The model under review builds one solid part; all positions refer to its coordinate system, in mm. Round coordinates to 2 decimals unless told otherwise and drop trailing zeros. Order: outer loops, then holes, each group sorted by start corner. A loop starts at its lowest first (then second) coordinate and runs counter-clockwise, first axis right, second up.
```python
from build123d import *

# Parameters (mm, degrees)
SKETCH1_W                                            = 150
SKETCH1_H                                            = 65
BOSS_EXTRUDE1_DEPTH                                  = 3
SKETCH2_W                                            = 130
SKETCH2_H                                            = 45
CUT_EXTRUDE1_DEPTH                                   = 82.793948431
FILLET1_R                                            = 2
SKETCH3_W                                            = 145
SKETCH3_H                                            = 60
CUT_EXTRUDE2_DEPTH                                   = 0.6
FILLET2_R                                            = 2
CSK_FOR_M2_5_CROSS_RECESSED_CTSK_HEAD_WO_D           = 2.7
CSK_FOR_M2_5_CROSS_RECESSED_CTSK_HEAD_WO_CSINK_D     = 5.4
CSK_FOR_M2_5_CROSS_RECESSED_CTSK_HEAD_WO_CSINK_ANGLE = 90
CHAMFER1_SIZE                                        = 1


with BuildPart() as part:
    # Sketch1 → Boss-Extrude1 (new body)
    with BuildSketch(Plane.XY):
        Rectangle(SKETCH1_W, SKETCH1_H)
    extrude(amount=BOSS_EXTRUDE1_DEPTH)

    # Sketch2 → Cut-Extrude1 (cut, through all)
    with BuildSketch(Plane.XY.offset(3)):
        Rectangle(SKETCH2_W, SKETCH2_H)
    extrude(amount=-CUT_EXTRUDE1_DEPTH, mode=Mode.SUBTRACT)

    # Fillet1
    fillet1_edges = [part.edges().sort_by_distance(p)[0] for p in [
        (-65, -22.5, 1.5),
        (-65, 22.5, 1.5),
        (65, 22.5, 1.5),
        (65, -22.5, 1.5),
        (-75, 32.5, 1.5),
        (75, 32.5, 1.5),
        (75, -32.5, 1.5),
        (-75, -32.5, 1.5),
    ]]
    fillet(fillet1_edges, radius=FILLET1_R)

    # Sketch3 → Cut-Extrude2 (cut)
    with BuildSketch(Plane.XY):
        Rectangle(SKETCH3_W, SKETCH3_H)
    extrude(amount=CUT_EXTRUDE2_DEPTH, mode=Mode.SUBTRACT)

    # Fillet2
    fillet2_edges = [part.edges().sort_by_distance(p)[0] for p in [
        (-72.5, 30, 0.3),
        (-72.5, -30, 0.3),
        (72.5, -30, 0.3),
        (72.5, 30, 0.3),
    ]]
    fillet(fillet2_edges, radius=FILLET2_R)

    # CSK for M2.5 Cross recessed CTSK head wood screws1 (through all)
    with Locations(Plane.XY.offset(3)):
        with Locations((-70, 27.5), (-70, 17.5), (-70, 5.833333333), (-70, -5.833333333), (-70, -17.5), (-70, -27.5), (-60, 27.5), (-42.857142857, 27.5), (-25.714285714, 27.5), (-8.571428571, 27.5), (8.571428571, 27.5), (25.714285714, 27.5), (42.857142857, 27.5), (60, 27.5), (70, 27.5), (70, 17.5), (70, 5.833333333), (70, -5.833333333), (70, -17.5), (70, -27.5), (60, -27.5), (42.857142857, -27.5), (25.714285714, -27.5), (8.571428571, -27.5), (-8.571428571, -27.5), (-25.714285714, -27.5), (-42.857142857, -27.5), (-60, -27.5)):
            CounterSinkHole(CSK_FOR_M2_5_CROSS_RECESSED_CTSK_HEAD_WO_D / 2, CSK_FOR_M2_5_CROSS_RECESSED_CTSK_HEAD_WO_CSINK_D / 2, counter_sink_angle=CSK_FOR_M2_5_CROSS_RECESSED_CTSK_HEAD_WO_CSINK_ANGLE)

    # Chamfer1
    chamfer1_edges = [part.edges().sort_by_distance(p)[0] for p in [
        (0, 32.5, 3),
        (75, 0, 3),
        (-75, 0, 3),
        (0, -32.5, 3),
        (-74.414213562, 31.914213562, 3),
        (-74.414213562, -31.914213562, 3),
        (74.414213562, -31.914213562, 3),
        (74.414213562, 31.914213562, 3),
    ]]
    chamfer(chamfer1_edges, length=CHAMFER1_SIZE)


solid = part.part
```
(1) To check wall thickness, follow probe 1 along X at (y, z) = (-17.5, 1.55); probe 2 along Y at (x, z) = (-25.5, 1.7); probe 3 along Y at (x, z) = (-43, 1.5). State the ranges of each line that lie inside material, in increasing order.
Data:
probe 1: x = -75 to -71.35, -68.65 to -65, 65 to 68.65, 71.35 to 75
probe 2: y = -32.5 to -28.88, -26.12 to -22.5, 22.5 to 26.12, 28.88 to 32.5
probe 3: y = -32.5 to -28.84, -26.16 to -22.5, 22.5 to 26.16, 28.84 to 32.5
(2) Draft analysis for pull direction X (two halves, no side actions). For faces 1 (the cylindrical face through (-43.48, -28.698, 1.118)), 2 (the cylindrical face through (69.38, 26.3, 1.12)), 3 (the flat face through (-6, 23, 3)), state which applies: pulls with the +X half, pulls with the -X half, needs draft (parallel to the pull), parting line crosses it, or undercut.
Data:
face 1: undercut
face 2: undercut
face 3: needs draft
(3) Consider section B-B (x = 60). Write out the cut boundary in (y, z).
Data:
outline: (-32.5, 0) - (-30, 0) - (-30, 0.6) - (-28.85, 0.6) - (-28.85, 1.65) - (-30.2, 3) - (-31.5, 3) - (-32.5, 2) - close; (-26.15, 0.6) - (-22.5, 0.6) - (-22.5, 3) - (-24.8, 3) - (-26.15, 1.65) - close; (22.5, 0.6) - (26.15, 0.6) - (26.15, 1.65) - (24.8, 3) - (22.5, 3) - close; (28.85, 0.6) - (30, 0.6) - (30, 0) - (32.5, 0) - (32.5, 2) - (31.5, 3) - (30.2, 3) - (28.85, 1.65) - close
(4) Consider section D-D (x = -31). Write out the cut boundary in (y, z), and give its area (3 significant figures).
Data:
outline: (-32.5, 0) - (-30, 0) - (-30, 0.6) - (-22.5, 0.6) - (-22.5, 3) - (-31.5, 3) - (-32.5, 2) - close; (22.5, 0.6) - (30, 0.6) - (30, 0) - (32.5, 0) - (32.5, 2) - (31.5, 3) - (22.5, 3) - close
area: 50.0 mm2
(5) Insertion check: pin 1 (3 mm diameter, centred on x = 70, y = 27.5, fed in from +Z); pin 2 (4.5 mm diameter, centred on x = -70, y = -27.5, fed in from +Z); pin 3 (4.5 mm diameter, centred on x = -70, y = 17.5, fed in from -Z); pin 4 (1.6 mm diameter, centred on x = -70, y = -17.5, fed in from +Z). Each pin has a flat end and moves straight along its axis. Give the tip position at first contact, or say it passes through.
Data:
pin 1: stops at z = 1.8
pin 2: stops at z = 2.55
pin 3: stops at z = 0.6
pin 4: passes through
(6) Consider section A-A (y = 17.5). Write out the cut boundary in (x, z), and give its area (3 significant figures).
Data:
outline: (-75, 0) - (-72.5, 0) - (-72.5, 0.6) - (-71.35, 0.6) - (-71.35, 1.65) - (-72.7, 3) - (-74, 3) - (-75, 2) - close; (-68.65, 0.6) - (-65, 0.6) - (-65, 3) - (-67.3, 3) - (-68.65, 1.65) - close; (65, 0.6) - (68.65, 0.6) - (68.65, 1.65) - (67.3, 3) - (65, 3) - close; (71.35, 0.6) - (72.5, 0.6) - (72.5, 0) - (75, 0) - (75, 2) - (74, 3) - (72.7, 3) - (71.35, 1.65) - close
area: 33.4 mm2
(7) Consider section C-C (y = -10). Write out the cut boundary in (x, z).
Data:
outline: (-75, 0) - (-72.5, 0) - (-72.5, 0.6) - (-65, 0.6) - (-65, 3) - (-74, 3) - (-75, 2) - close; (65, 0.6) - (72.5, 0.6) - (72.5, 0) - (75, 0) - (75, 2) - (74, 3) - (65, 3) - close
